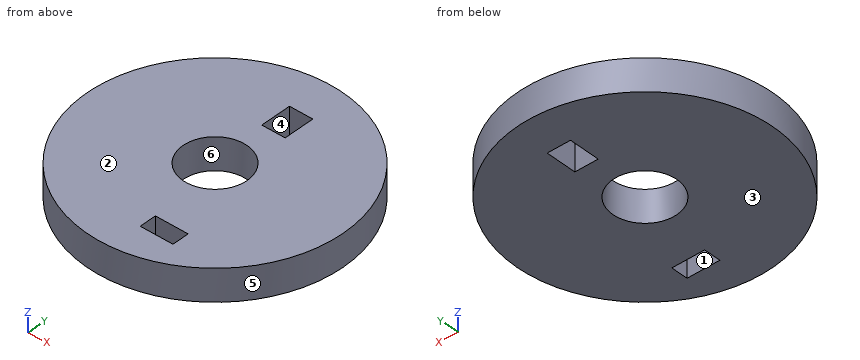
```python
from build123d import *

# Parameters (mm, degrees)
F0_R     = 50.8
F0_R_2   = 12.7
F0_W     = 13.006554
F0_H     = 6.700346
F0_W_2   = 9.262241
F0_H_2   = 12.218274
F1_DEPTH = 6.35


with BuildPart() as f1:
    # F0 (on Top) → F1 (new body, symmetric)
    with BuildSketch(Plane.XY):
        Circle(F0_R)
        Circle(F0_R_2, mode=Mode.SUBTRACT)
        with Locations((10.444656, -34.092932)):
            Rectangle(F0_W, F0_H, mode=Mode.SUBTRACT)
        with Locations((2.66043, 28.969139)):
            Rectangle(F0_W_2, F0_H_2, mode=Mode.SUBTRACT)
    extrude(amount=F1_DEPTH, both=True)


solid = f1.part
```
Geometry: final body of the model. Coordinates: model frame, mm. Face numbers are marked on the shaded views. A direction names the side the tool comes from. Round coordinates to 2 decimals unless told otherwise and drop trailing zeros. Order: outer loops, then holes, each group sorted by start corner. A loop starts at its lowest first (then second) coordinate and runs counter-clockwise, first axis right, second up. Notation, with made-up numbers: M -10.75,42.5 L -2.75,42.5 A32 cw -2.75,73.5 Z; hole C -19,75.5 d3. An arc over 180 degrees is marked long. One line per item, written item: value.
(1) Cut plane A-A (y = 0). Return the cut outline in (x, z).
Result sheet:
outline: M -50.8,-6.35 L -12.7,-6.35 L -12.7,6.35 L -50.8,6.35 Z; M 12.7,-6.35 L 50.8,-6.35 L 50.8,6.35 L 12.7,6.35 Z
(2) Line query: probe 1 along Y at (x, z) = (0, 2.5); probe 2 along Y at (x, z) = (7.5, 1.25); probe 3 along X at (y, z) = (-8.5, -3.5). Output: solid intervals per line, ascending. Write a range as [from, to].
Result sheet:
probe 1: [-50.8, -12.7], [12.7, 22.86], [35.08, 50.8]
probe 2: [-50.24, -37.44], [-30.74, -10.25], [10.25, 50.24]
probe 3: [-50.08, -9.44], [9.44, 50.08]
(3) Cut plane B-B (x = 0). Return the cut outline in (y, z).
Result sheet:
outline: M -50.8,-6.35 L -12.7,-6.35 L -12.7,6.35 L -50.8,6.35 Z; M 12.7,-6.35 L 22.86,-6.35 L 22.86,6.35 L 12.7,6.35 Z; M 35.08,-6.35 L 50.8,-6.35 L 50.8,6.35 L 35.08,6.35 Z
(4) Cut plane C-C (z = 1.5). Return the cut outline in (x, y), and give its area (3 significant figures).
Result sheet:
outline: C 0,0 d101.6; hole C 0,0 d25.4; hole M -1.97,22.86 L 7.29,22.86 L 7.29,35.08 L -1.97,35.08 Z; hole M 3.94,-37.44 L 16.95,-37.44 L 16.95,-30.74 L 3.94,-30.74 Z
area: 7,400 mm2
(5) Pin query (flat end, axial travel): P1, Ø7.5, axis at x = 4.5, z = -2.5, coming from the -Y side; P2, Ø1, axis at x = -25, z = 4, coming from the +Y side; P3, Ø2, axis at x = 20.5, z = -2, coming from the -Y side; P4, Ø23, axis at x = 0, y = 0, coming from the -Z side. Return the tip coordinate at first contact, or that it passes through.
Result sheet:
P1: y = -50.79
P2: y = 44.5
P3: y = -46.91
P4: through
(6) Cut plane D-D (x = 15). Return the cut outline in (y, z).
Result sheet:
outline: M -48.53,-6.35 L -37.44,-6.35 L -37.44,6.35 L -48.53,6.35 Z; M -30.74,-6.35 L 48.53,-6.35 L 48.53,6.35 L -30.74,6.35 Z
(7) Pull-direction query (Y, two-part tool) for the marked faces 3, 4, 5 and 6; classes: pulls with the +Y half, pulls with the -Y half, needs draft (parallel to the pull), parting line crosses it, or undercut.
Result sheet:
face 3: needs draft
face 4: undercut
face 5: parting line crosses it
face 6: undercut
(8) Reachability of the marked faces 1 and 2 from +Z, -Z, +X, -X, +Y, -Y: full face, straight path, thin tool, end or side. Return the list, or none.
Result sheet:
face 1: +Z, -Z
face 2: +Z, +X, -X, +Y, -Y
